Could you check a few things on this drawing? It's one solid part, dimensions in mm from its lowest x, y, z. A direction names the side the tool comes from. Give positions to 0.01 mm unless a question says otherwise; leave off trailing zeros. Order: outer loops, then holes, each group sorted by start corner. A loop starts at its lowest first (then second) coordinate and runs counter-clockwise, first axis right, second up.
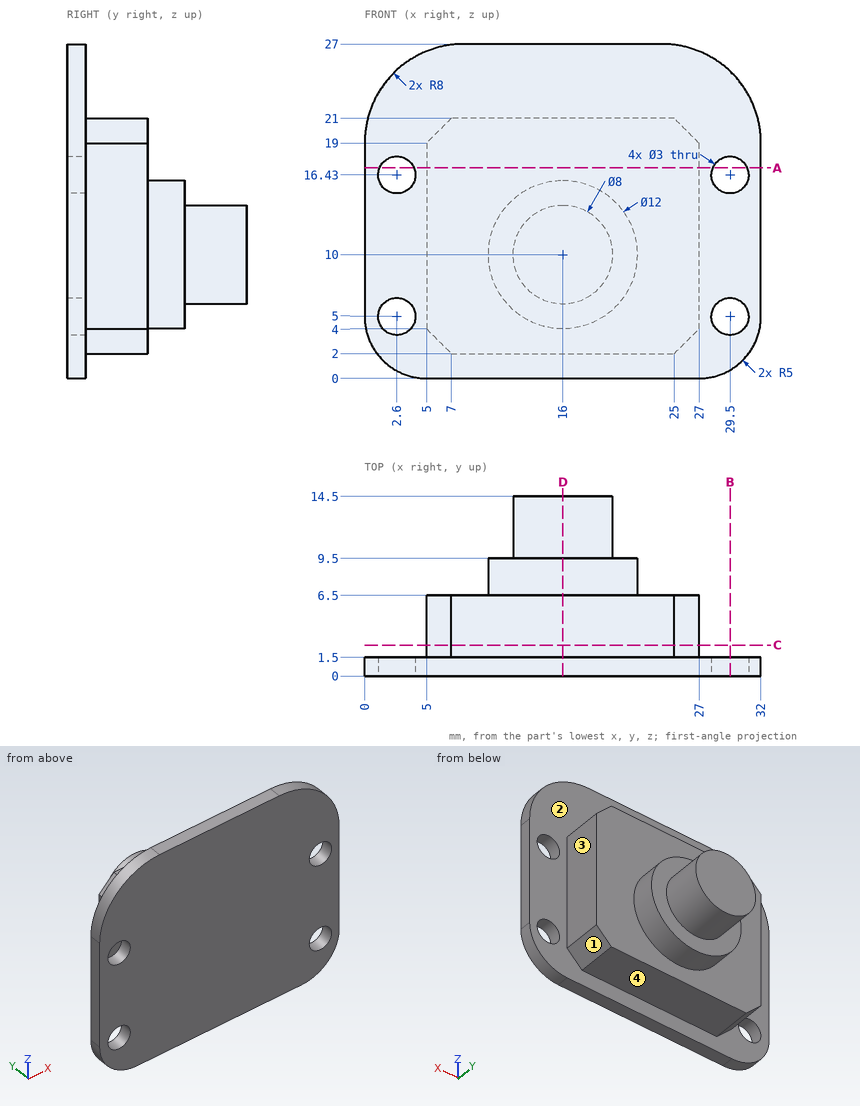
1) I'm going to push flat-ended pins straight in: pin 1 Ø3 at (x, y) = (11.5, 9.5) entering from -Z; pin 2 Ø12 at (x, z) = (8, 22) entering from +Y; pin 3 Ø1 at (x, y) = (11, 8.5) entering from -Z. Where does each tip first touch, or does it pass through?
2) Suppose I cut it at C-C (y = 2.5). Please give me the cut outline in (x, z).
3) If I drill on line 1 (X direction, y = 0.6, z = 5); line 2 (Y direction, x = 6, z = 9.75); line 3 (Y direction, x = 20, z = 13), over which ranges is the centre line in solid material (lowest first)?
4) Which directions (+Z, -Z, +X, -X, +Y, -Y) give clear straight access to the entire face, cutting with the end or side of a thin tool? Please do the marked faces 1, 2, 3 and 4.
5) Suppose I cut it at D-D (x = 16). Please give me the cut outline in (y, z).
6) Suppose I cut it at B-B (x = 29.5). Please give me the cut outline in (y, z).
7) Suppose I cut it at A-A (z = 17). Please give me the cut outline in (x, y).
Results:
1. pin 1: stops at z = 4.8
1. pin 2: stops at y = 6.5
1. pin 3: stops at z = 6.03
2. outline: (5, 4) - (7, 2) - (25, 2) - (27, 4) - (27, 19) - (25, 21) - (7, 21) - (5, 19) - close
3. line 1: x = 0 to 1.1, 4.1 to 28, 31 to 32
3. line 2: y = 0 to 6.5
3. line 3: y = 0 to 9.5
4. face 1: -Z, +X, +Y
4. face 2: +Y
4. face 3: +Z, -Z, +X, +Y
4. face 4: -Z, +X, -X, +Y
5. outline: (0, 0) - (1.5, 0) - (1.5, 2) - (6.5, 2) - (6.5, 4) - (9.5, 4) - (9.5, 6) - (14.5, 6) - (14.5, 14) - (9.5, 14) - (9.5, 16) - (6.5, 16) - (6.5, 21) - (1.5, 21) - (1.5, 27) - (0, 27) - close
6. outline: (0, 0.67) - (1.5, 0.67) - (1.5, 3.5) - (0, 3.5) - close; (0, 6.5) - (1.5, 6.5) - (1.5, 14.93) - (0, 14.93) - close; (0, 17.93) - (1.5, 17.93) - (1.5, 24.81) - (0, 24.81) - close
7. outline: (0, 0) - (1.21, 0) - (1.21, 1.5) - (0, 1.5) - close; (3.99, 0) - (28.11, 0) - (28.11, 1.5) - (27, 1.5) - (27, 6.5) - (5, 6.5) - (5, 1.5) - (3.99, 1.5) - close; (30.89, 0) - (32, 0) - (32, 1.5) - (30.89, 1.5) - close
